Design review of the part built by this model. Coordinates are the model's own, in mm. A direction names the side the tool comes from. Give positions to 0.01 mm unless a question says otherwise; leave off trailing zeros. Order: outer loops, then holes, each group sorted by start corner. A loop starts at its lowest first (then second) coordinate and runs counter-clockwise, first axis right, second up. Notation, with made-up numbers: (35, 70.25) -> (54, 70.25) arc R26 ccw to (54, 91.25) -> close; hole circle Ø1 at (48, 70.25). An arc over 180 degrees is marked (long way). Return JSON: item names as keys, results as strings.
```python
from build123d import *

# Parameters (mm, degrees)
SKETCH1_R           = 1.905
SKETCH1_R_2         = 6.985
BOSS_EXTRUDE1_DEPTH = 12.7
FILLET1_R           = 2.54
SKETCH2_R           = 3.175
CUT_EXTRUDE1_DEPTH  = 7.35


with BuildPart() as part:
    # Sketch1 → Boss-Extrude1 (new body)
    with BuildSketch(Plane(origin=(0, 0, 0), x_dir=(1, 0, 0), z_dir=(0, 1, 0))):
        Polygon((-25.4, 0), (12.7, 0), (12.7, 6.35), (0, 6.35), (0, 25.4), (-25.4, 25.4), align=None)
        with Locations((-17.4625, 4.451108029)):
            Circle(SKETCH1_R, mode=Mode.SUBTRACT)
        with Locations((-3.175, 12.7)):
            Circle(SKETCH1_R, mode=Mode.SUBTRACT)
        with Locations((-12.7, 12.7)):
            Circle(SKETCH1_R_2, mode=Mode.SUBTRACT)
        with Locations((-17.4625, 20.948891971)):
            Circle(SKETCH1_R, mode=Mode.SUBTRACT)
    extrude(amount=BOSS_EXTRUDE1_DEPTH)

    # Fillet1
    fillet1_edges = [part.edges().sort_by_distance(p)[0] for p in [
        (0, 6.35, -6.35),
        (0, 6.35, -25.4),
        (-25.4, 6.35, -25.4),
        (-25.4, 6.35, 0),
    ]]
    fillet(fillet1_edges, radius=FILLET1_R)

    # Sketch2 → Cut-Extrude1 (cut, through all)
    with BuildSketch(Plane(origin=(0, 0, -6.35), x_dir=(-1, 0, 0), z_dir=(0, 0, -1))):
        with Locations((-7.62, 6.35)):
            Circle(SKETCH2_R)
    extrude(amount=-CUT_EXTRUDE1_DEPTH, mode=Mode.SUBTRACT)


solid = part.part
```
Item 1: Add section A-A (x = 7.62). Give the boundary of the cut face in (y, z) (3 decimals).
Result set:
{"outline": "(0, -6.35) -> (3.175, -6.35) -> (3.175, 0) -> (0, 0) -> close; (9.525, -6.35) -> (12.7, -6.35) -> (12.7, 0) -> (9.525, 0) -> close"}
Item 2: Add section C-C (z = -12.7). Give the boundary of the cut face in (x, y) (3 decimals).
Result set:
{"outline": "(-25.4, 0) -> (-19.685, 0) -> (-19.685, 12.7) -> (-25.4, 12.7) -> close; (-5.715, 0) -> (-5.08, 0) -> (-5.08, 12.7) -> (-5.715, 12.7) -> close; (-1.27, 0) -> (0, 0) -> (0, 12.7) -> (-1.27, 12.7) -> close"}
Item 3: For pin 1 (2 mm diameter, centred on y = 7.5, z = -9.5, fed in from +X); pin 2 (8 mm diameter, centred on x = -9, z = -7, fed in from +Y), all flat-tipped, find the tip position at first contact; note any pin that passes through.
Result set:
{"pin 1": "stops at x = 0.03", "pin 2": "stops at y = 12.7"}
Item 4: Add section D-D (z = -4). Give the boundary of the cut face in (x, y) (3 decimals).
Result set:
{"outline": "(-25.4, 0) -> (-19.313, 0) -> (-19.313, 12.7) -> (-25.4, 12.7) -> close; (-15.612, 0) -> (12.7, 0) -> (12.7, 12.7) -> (-15.612, 12.7) -> close; hole circle Ø6.35 at (7.62, 6.35)"}
Item 5: Add section B-B (y = 5.75). Give the number of separate pieces and of enclosed holes in the cut face, plus the area to 3 significant figures.
Result set:
{"separate pieces": "2", "enclosed holes": "4", "area": "496 mm^2"}
Item 6: Mouldability with a two-part tool opening along Z and no side actions: class faces 1 (the face through (-0.764, 6.439, -24.676)), 2 (the face through (12.7, 6, -3)), 3 (the face through (-19.366, 6.261, -21.033)), 4 (the face through (-5, 6, 0)) as released by +Z, released by -Z, zero draft, split by the parting line, or undercut.
Result set:
{"face 1": "released by -Z", "face 2": "zero draft", "face 3": "undercut", "face 4": "released by +Z"}
Item 7: Machinability: for faces 5 (the face through (-13, 6, -25.4)), 6 (the face through (0, 6, -16)), which of the approach directions +Z, -Z, +X, -X, +Y, -Y give a long, thin tool a straight path to every point of the face, cutting with its end or side? Answer none if there is none.
Result set:
{"face 5": "-Z, +X, -X, +Y, -Y", "face 6": "-Z, +X, +Y, -Y"}
Item 8: Wall thickness on L1, parallel to Y at x = 7.62, z = -3.5 (3 decimals); L2, parallel to Z at x = -12.7, y = 9.5 (3 decimals); L3, parallel to X at y = 2.25, z = -14.25: over which ranges is each line inside the solid? List them lowest first. Write a range as [from, to].
Result set:
{"L1": "y = [0, 3.175], [9.525, 12.7]", "L2": "z = [-25.4, -19.685], [-5.715, 0]", "L3": "x = [-25.4, -19.51], [-5.89, -4.28], [-2.07, 0]"}
